```python
from build123d import *

# Parameters (mm, degrees)
BOSS_EXTRUDE1_DEPTH = 63.5
SKETCH3_R           = 1.5
CUT_EXTRUDE1_DEPTH  = 86.194189943
SKETCH3_3_R         = 1.5
BOSS_EXTRUDE2_DEPTH = 3.175
CUT_EXTRUDE2_DEPTH  = 86.194189943
CUT_EXTRUDE3_DEPTH  = 3.175
SKETCH6_W           = 25.4
SKETCH6_H           = 17.35
BOSS_EXTRUDE3_DEPTH = 1
BOSS_EXTRUDE4_START = -1
SKETCH6_3_W         = 25.4
SKETCH6_3_H         = 23.35
SKETCH6_3_W_2       = 20.55
SKETCH6_3_H_2       = 13.35
BOSS_EXTRUDE4_DEPTH = 7
CUT_EXTRUDE4_DEPTH  = 73.122136159
SKETCH6_4_W         = 25.4
SKETCH6_4_H         = 6
BOSS_EXTRUDE5_DEPTH = 3.175
FILLET2_R           = 5


with BuildPart() as part:
    # Sketch2 → Boss-Extrude1 (new body)
    with BuildSketch(Plane(origin=(0, 0, 0), x_dir=(0, 0, -1), z_dir=(1, 0, 0))):
        Polygon((-50.8, 0), (0, 0), (0, 25.4), (-4.7625, 25.4), (-4.7625, 3.175), (-50.8, 3.175), align=None)
    extrude(amount=BOSS_EXTRUDE1_DEPTH)

    # Sketch3 → Cut-Extrude1 (cut, through all)
    with BuildSketch(Plane(origin=(0, 0, 0), x_dir=(-1, 0, 0), z_dir=(0, 0, -1))):
        with Locations(Location((-12.7, 12.7, 0), (0, 0, 90))):
            Circle(SKETCH3_R)
    extrude(amount=-CUT_EXTRUDE1_DEPTH, mode=Mode.SUBTRACT)

    # Sketch3<3> → Boss-Extrude2 (add)
    with BuildSketch(Plane(origin=(0, 0, 0), x_dir=(-1, 0, 0), z_dir=(0, 0, -1))):
        with Locations(Location((-50.8, 12.7, 0), (0, 0, 180))):
            Circle(SKETCH3_3_R)
    extrude(amount=BOSS_EXTRUDE2_DEPTH)

    # Sketch4 → Cut-Extrude2 (cut, through all)
    with BuildSketch(Plane(origin=(0, 0, 0), x_dir=(-1, 0, 0), z_dir=(0, 0, -1))):
        with BuildLine():
            Line((-63.5, 25.4), (-63.5, 0))
            ThreePointArc((-63.5, 0), (-52.079919454, 18.268649317), (-31.75, 25.4))
            Line((-31.75, 25.4), (-63.5, 25.4))
        make_face()
        with BuildLine():
            ThreePointArc((-31.75, 25.4), (-11.420080546, 18.268649317), (0, 0))
            Line((0, 0), (0, 25.4))
            Line((0, 25.4), (-31.75, 25.4))
        make_face()
    extrude(amount=-CUT_EXTRUDE2_DEPTH, mode=Mode.SUBTRACT)

    # Sketch5 → Cut-Extrude3 (cut)
    with BuildSketch(Plane(origin=(0, 3.175, 0), x_dir=(1, 0, 0), z_dir=(0, 1, 0))):
        with BuildLine():
            Line((44.45, -4.7625), (19.05, -4.7625))
            Line((19.05, -4.7625), (19.05, -41.275))
            ThreePointArc((19.05, -41.275), (16.260192091, -48.010192091), (9.525, -50.8))
            Line((9.525, -50.8), (53.975, -50.8))
            ThreePointArc((53.975, -50.8), (47.239807909, -48.010192091), (44.45, -41.275))
            Line((44.45, -41.275), (44.45, -4.7625))
        make_face()
        with BuildLine():
            ThreePointArc((9.525, -50.8), (4.400279527, -49.303876949), (0.885472424, -45.285509726))
            Line((0.885472424, -45.285509726), (0.885472424, -50.8))
            Line((0.885472424, -50.8), (9.525, -50.8))
        make_face()
        with BuildLine():
            ThreePointArc((0.885472424, -45.285509726), (0.224002065, -43.328548738), (0, -41.275))
            Line((0, -41.275), (0, -50.8))
            Line((0, -50.8), (0.885472424, -50.8))
            Line((0.885472424, -50.8), (0.885472424, -45.285509726))
        make_face()
        with BuildLine():
            ThreePointArc((62.614527576, -45.285509726), (59.099720473, -49.303876949), (53.975, -50.8))
            Line((53.975, -50.8), (62.614527576, -50.8))
            Line((62.614527576, -50.8), (62.614527576, -45.285509726))
        make_face()
        with BuildLine():
            ThreePointArc((63.5, -41.275), (63.275997935, -43.328548738), (62.614527576, -45.285509726))
            Line((62.614527576, -45.285509726), (62.614527576, -50.8))
            Line((62.614527576, -50.8), (63.5, -50.8))
            Line((63.5, -50.8), (63.5, -41.275))
        make_face()
    extrude(amount=-CUT_EXTRUDE3_DEPTH, mode=Mode.SUBTRACT)

    # Sketch6 → Boss-Extrude3 (add)
    with BuildSketch(Plane.XZ):
        with Locations((31.75, 19.4375)):
            Rectangle(SKETCH6_W, SKETCH6_H)
    extrude(amount=-BOSS_EXTRUDE3_DEPTH)

    # Sketch6<3> → Boss-Extrude4 (add)
    with BuildSketch(Plane.XZ.offset(BOSS_EXTRUDE4_START)):
        with Locations((31.75, 16.4375)):
            Rectangle(SKETCH6_3_W, SKETCH6_3_H)
        with Locations((31.75, 19.4375)):
            Rectangle(SKETCH6_3_W_2, SKETCH6_3_H_2, mode=Mode.SUBTRACT)
    extrude(amount=-BOSS_EXTRUDE4_DEPTH)

    # Sketch7 → Cut-Extrude4 (cut, through all)
    with BuildSketch(Plane.ZY.offset(-19.05)):
        Polygon((10.7625, 8), (28.1125, 8), (28.1125, 4.5), align=None)
    extrude(amount=-CUT_EXTRUDE4_DEPTH, mode=Mode.SUBTRACT)

    # Sketch6<4> → Boss-Extrude5 (add)
    with BuildSketch(Plane.XZ):
        with Locations((31.75, 7.7625)):
            Rectangle(SKETCH6_4_W, SKETCH6_4_H)
    extrude(amount=-BOSS_EXTRUDE5_DEPTH)

    # Fillet2
    fillet2_edges = [part.edges().sort_by_distance(p)[0] for p in [
        (9.967736212, 3.175, 4.7625),
    ]]
    fillet(fillet2_edges, radius=FILLET2_R)


solid = part.part
```
Here's how the part is built. I have some questions about the finished solid (model axes, mm). A direction names the side the tool comes from. Coordinates: 2 decimals unless noted, no trailing zeros. Write each loop counter-clockwise with the first axis right and the second up, starting at its lowest first coordinate (ties: lowest second). Pieces come first, ordered by that corner, then holes. Notation, with made-up numbers: M -38,84.25 L 4,84.25 A32 cw 4,117.25 Z; hole C 60,87.5 d9. An arc over 180 degrees is marked long. Answer as CSV lines item,"result". Start each with the question number.
Q1. If we mould it in two halves opening along X, with no side actions, what happens to faces 4 (the cylindrical face through (11.37, 13.39, 2.35)), 5 (the flat face through (44.45, 5, 14)), 6 (the flat face through (32, 8, 8))? For each: pulls with the +X half, pulls with the -X half, needs draft (parallel to the pull), parting line crosses it, or undercut.
Q2. Will these pins go through, and if not, where does the flat tip stop? pin 1 Ø9 at (x, z) = (7, 27.5) entering from +Y (3 decimals); pin 2 Ø1.4 at (y, z) = (6, 17) entering from -X; pin 3 Ø8.5 at (x, y) = (24.5, 17) entering from +Z; pin 4 Ø2.5 at (x, y) = (12.7, 12.7) entering from +Z.
Q3. Suppose I cut it at C-C, the plane x = 12.7. List the corners of the cut face in (y, z) for me (1 decimal).
Q4. Suppose I cut it at D-D, the plane x = 50.8. List the corners of the cut face in (y, z) for me (1 decimal), then the cut area to 3 significant figures.
Q5. Suppose I cut it at B-B, the plane y = 12.7. List the corners of the cut face in (x, z) for me (1 decimal), then the cut area to 3 significant figures.
Q6. I need wall thicknesses on probe 1 along Z at (x, y) = (29.5, 5); probe 2 along Z at (x, y) = (19, 9.75); probe 3 along X at (y, z) = (3.25, 25) (3 decimals). Which ranges of each line are inside material? Lowest first, please. Write a range as [from, to].
Q7. For faces 1 (the flat face through (21.475, 4, 19)), 2 (the flat face through (19.05, 5, 14)), 3 (the cylindrical face through (52.186, 13.275, -1.565)), which set-ups out of +Z, -Z, +X, -X, +Y, -Y let a thin tool reach every point of the face, with its end or its side?
Entries:
1,face 4,"undercut"
1,face 5,"pulls with the +X half"
1,face 6,"needs draft"
2,pin 1,"stops at y = 3.175"
2,pin 2,"stops at x = 19.05"
2,pin 3,"stops at z = 4.76"
2,pin 4,"passes through"
3,outline,"M 0,0 L 11.2,0 L 11.2,4.8 L 8.2,4.8 A5 cw 3.2,9.8 L 3.2,50.3 L 0,50.3 Z; M 14.2,0 L 19.2,0 L 19.2,4.8 L 14.2,4.8 Z"
4,outline,"M 0,0 L 11.2,0 L 11.2,-3.2 L 14.2,-3.2 L 14.2,0 L 19.2,0 L 19.2,4.8 L 8.2,4.8 A5 cw 3.2,9.8 L 3.2,50.3 L 0,50.3 Z"
4,area,"251 mm²"
5,outline,"M 6,0 L 11.2,0 L 11.2,4.8 L 6,4.8 Z; M 14.2,0 L 49.3,0 L 49.3,-3.2 L 52.3,-3.2 L 52.3,0 L 57.5,0 L 57.5,4.8 L 14.2,4.8 Z"
5,area,"241 mm²"
6,probe 1,"z = [0, 12.76]"
6,probe 2,"z = [0, 4.76]"
6,probe 3,"x = [19.05, 21.475], [42.025, 44.45]"
7,face 1,"+Y"
7,face 2,"+Z, -X, +Y"
7,face 3,"-Z"
